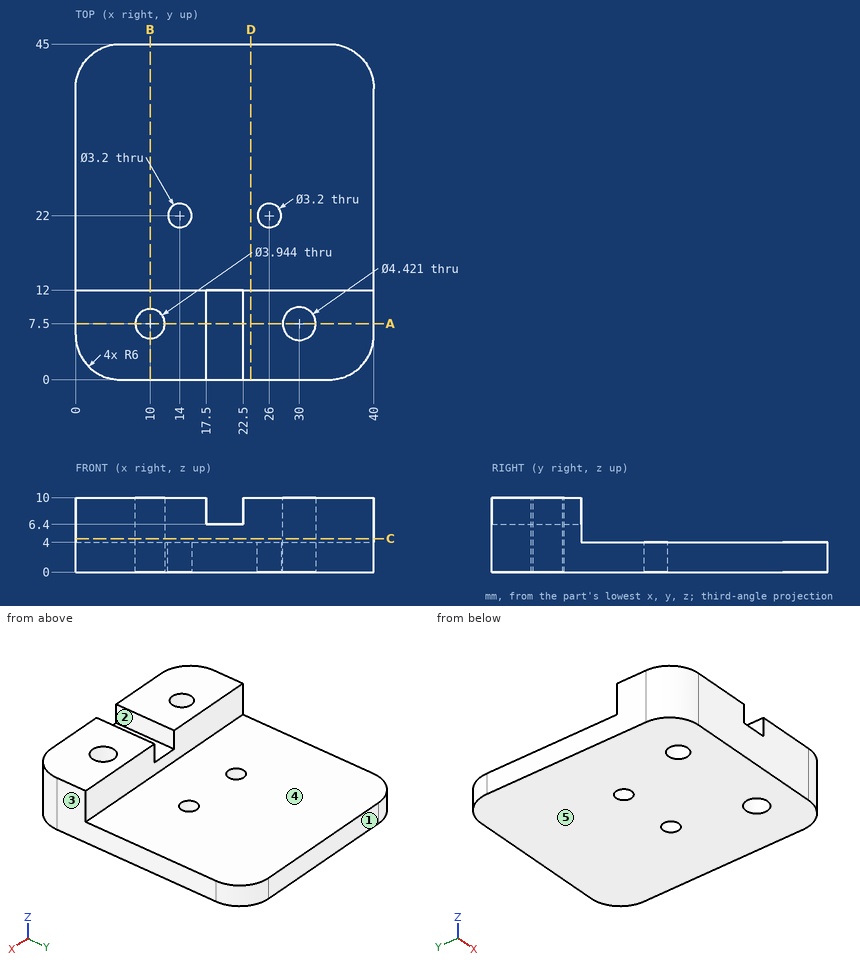
The figure shows three views and two pictorial views of one solid part (mm, origin at its lowest corner). Answer the questions. A direction names the side the tool comes from. Coordinates: 2 decimals unless noted, no trailing zeros. Loops run counter-clockwise (first coordinate to the right, second up) from the corner with the lowest first, then second, coordinate; pieces in that order, holes last.
1) A tool of negligible diameter and unlimited length cuts with its end or side. For the marked faces 4 and 5, from which of +Z, -Z, +X, -X, +Y, -Y can it reach the whole face along a straight path? Write none if from no direction.
2) Find the intervals of material crossed by L1, parallel to Y at x = 29, z = 7.75; L2, parallel to Y at x = 14, z = 2; L3, parallel to X at y = 6.5, z = 1, in increasing order.
3) Flat-ended cylindrical pins translate along their axes: pin 1 Ø2.5 at (x, y) = (19.5, 5.5) entering from +Z; pin 2 Ø4 at (x, z) = (14, 6.5) entering from +Y; pin 3 Ø4 at (x, y) = (14.5, 33) entering from +Z. Find the tip coordinate at first contact, or state that the pin passes through.
4) Find section C-C on z = 4.5. Write down the section's boundary in (x, y), then the cut area to 3 significant figures.
5) Find section B-B on x = 10. Write down the section's boundary in (y, z).
6) Determine the mould class of the marked faces 1, 2 and 3 for opening direction X: pulls with the +X half, pulls with the -X half, needs draft (parallel to the pull), parting line crosses it, or undercut.
7) Find section D-D on x = 23.5. Write down the section's boundary in (y, z).
8) Find section A-A on y = 7.5. Write down the section's boundary in (x, z).
Values:
1. face 4: +Z, +X, -X, +Y
1. face 5: -Z, +X, -X, +Y, -Y
2. L1: y = 0 to 5.53, 9.47 to 12
2. L2: y = 0 to 20.4, 23.6 to 45
2. L3: x = 0 to 8.3, 11.7 to 28.03, 31.97 to 40
3. pin 1: stops at z = 6.4
3. pin 2: stops at y = 12
3. pin 3: stops at z = 4
4. outline: (0, 6) arc R6 ccw to (6, 0) - (34, 0) arc R6 ccw to (40, 6) - (40, 12) - (0, 12) - close; hole circle Ø3.94 at (10, 7.5); hole circle Ø4.42 at (30, 7.5)
4. area: 437 mm2
5. outline: (0, 0) - (5.53, 0) - (5.53, 10) - (0, 10) - close; (9.47, 0) - (45, 0) - (45, 4) - (12, 4) - (12, 10) - (9.47, 10) - close
6. face 1: needs draft
6. face 2: undercut
6. face 3: pulls with the +X half
7. outline: (0, 0) - (45, 0) - (45, 4) - (12, 4) - (12, 10) - (0, 10) - close
8. outline: (0, 0) - (8.03, 0) - (8.03, 10) - (0, 10) - close; (11.97, 0) - (27.79, 0) - (27.79, 10) - (22.5, 10) - (22.5, 6.4) - (17.5, 6.4) - (17.5, 10) - (11.97, 10) - close; (32.21, 0) - (40, 0) - (40, 10) - (32.21, 10) - close
